CAD build for the part. Positions are in the model's coordinates, mm. A direction names the side the tool comes from. Coordinates: 2 decimals unless noted, no trailing zeros. Loops run counter-clockwise (first coordinate to the right, second up) from the corner with the lowest first, then second, coordinate; pieces in that order, holes last. Notation, with made-up numbers: (-21.75, 82) -> (27.25, 82) arc R28 ccw to (27.25, 118) -> close; hole circle Ø5 at (-38.5, 41.5). An arc over 180 degrees is marked (long way). Write each question's results on one line, items separated by ' | '.
from build123d import *

# Parameters (mm, degrees)
SKETCH1_W           = 200
SKETCH1_H           = 43
BOSS_EXTRUDE1_DEPTH = 25
SKETCH2_W           = 80
SKETCH2_H           = 39
CUT_EXTRUDE1_DEPTH  = 23
SKETCH3_W           = 28
SKETCH3_H           = 14
BOSS_EXTRUDE2_DEPTH = 8
SKETCH4_W           = 14
SKETCH4_H           = 2
BOSS_EXTRUDE3_DEPTH = 2.5
SKETCH5_W           = 14
SKETCH5_H           = 2
BOSS_EXTRUDE4_DEPTH = 2.5
SKETCH6_R           = 1
CUT_EXTRUDE2_DEPTH  = 2
SKETCH7_W           = 116
SKETCH7_H           = 43
CUT_EXTRUDE3_DEPTH  = 23
SKETCH8_W           = 46.953712071
SKETCH8_H           = 43
SKETCH8_R           = 2.1
BOSS_EXTRUDE6_DEPTH = 8
SKETCH9_W           = 10
SKETCH9_H           = 2
CUT_EXTRUDE4_DEPTH  = 61
SKETCH10_W          = 46.769233888
SKETCH10_H          = 43
SKETCH10_R          = 2.1
BOSS_EXTRUDE7_DEPTH = 8
SKETCH11_W          = 3
SKETCH11_H          = 10
CUT_EXTRUDE5_DEPTH  = 8
FILLET1_R           = 15
FILLET2_R           = 15


with BuildPart() as part:
    # Sketch1 → Boss-Extrude1 (new body)
    with BuildSketch(Plane(origin=(0, 0, 0), x_dir=(1, 0, 0), z_dir=(0, 1, 0))):
        with Locations((100, 21.5)):
            Rectangle(SKETCH1_W, SKETCH1_H)
    extrude(amount=BOSS_EXTRUDE1_DEPTH)

    # Sketch2 → Cut-Extrude1 (cut)
    with BuildSketch(Plane(origin=(0, 25, 0), x_dir=(1, 0, 0), z_dir=(0, 1, 0))):
        with Locations((42, 21.5)):
            Rectangle(SKETCH2_W, SKETCH2_H)
    extrude(amount=-CUT_EXTRUDE1_DEPTH, mode=Mode.SUBTRACT)

    # Sketch3 → Boss-Extrude2 (add)
    with BuildSketch(Plane.XZ):
        with Locations((25.914586037, -21)):
            Rectangle(SKETCH3_W, SKETCH3_H)
    extrude(amount=BOSS_EXTRUDE2_DEPTH)

    # Sketch4 → Boss-Extrude3 (add)
    with BuildSketch(Plane(origin=(39.914586037, 0, 0), x_dir=(0, 0, -1), z_dir=(1, 0, 0))):
        with Locations((21, -7)):
            Rectangle(SKETCH4_W, SKETCH4_H)
    extrude(amount=BOSS_EXTRUDE3_DEPTH)

    # Sketch5 → Boss-Extrude4 (add)
    with BuildSketch(Plane.ZY.offset(-11.914586037)):
        with Locations((-21, -7)):
            Rectangle(SKETCH5_W, SKETCH5_H)
    extrude(amount=BOSS_EXTRUDE4_DEPTH)

    # Sketch6 → Cut-Extrude2 (cut)
    with BuildSketch(Plane.XZ):
        with Locations(Location((25.914586037, -37.49, 0), (0, 0, 270))):
            Circle(SKETCH6_R)
        with Locations(Location((28.914586037, -37.49, 0), (0, 0, 270))):
            Circle(SKETCH6_R)
        with Locations(Location((22.914586037, -37.49, 0), (0, 0, 270))):
            Circle(SKETCH6_R)
    extrude(amount=-CUT_EXTRUDE2_DEPTH, mode=Mode.SUBTRACT)

    # Sketch7 → Cut-Extrude3 (cut)
    with BuildSketch(Plane(origin=(0, 25, 0), x_dir=(1, 0, 0), z_dir=(0, 1, 0))):
        with Locations((142, 21.5)):
            Rectangle(SKETCH7_W, SKETCH7_H)
    extrude(amount=-CUT_EXTRUDE3_DEPTH, mode=Mode.SUBTRACT)

    # Sketch8 → Boss-Extrude6 (add)
    with BuildSketch(Plane(origin=(0, 2, 0), x_dir=(1, 0, 0), z_dir=(0, 1, 0))):
        with Locations((176.523143965, 21.5)):
            Rectangle(SKETCH8_W, SKETCH8_H)
        with BuildLine():
            Line((167.769501391, 39.672770255), (184.769501391, 39.672770255))
            Line((184.769501391, 39.672770255), (184.769501391, 34.969828795))
            ThreePointArc((184.769501391, 34.969828795), (187.225820525, 33.318614715), (189.368743796, 31.277073268))
            Line((189.368743796, 31.277073268), (192.70603487, 33.203859168))
            ThreePointArc((192.70603487, 33.203859168), (197.487123783, 31.922770255), (196.20603487, 27.141681341))
            Line((196.20603487, 27.141681341), (192.868743796, 25.214895441))
            ThreePointArc((192.868743796, 25.214895441), (193.542844178, 22.480194155), (193.769501391, 19.672770255))
            ThreePointArc((193.769501391, 19.672770255), (182.474872367, 3.309904642), (163.170258986, 8.068467242))
            Line((163.170258986, 8.068467242), (159.832967911, 6.141681341))
            ThreePointArc((159.832967911, 6.141681341), (155.051878998, 7.422770255), (156.332967911, 12.203859168))
            Line((156.332967911, 12.203859168), (159.670258986, 14.130645068))
            ThreePointArc((159.670258986, 14.130645068), (159.958128459, 26.012258646), (167.769501391, 34.969828795))
            Line((167.769501391, 34.969828795), (167.769501391, 39.672770255))
        make_face(mode=Mode.SUBTRACT)
        with BuildLine():
            Line((192.70603487, 33.203859168), (189.368743796, 31.277073268))
            ThreePointArc((189.368743796, 31.277073268), (191.424945957, 28.422770255), (192.868743796, 25.214895441))
            Line((192.868743796, 25.214895441), (196.20603487, 27.141681341))
            ThreePointArc((196.20603487, 27.141681341), (197.487123783, 31.922770255), (192.70603487, 33.203859168))
        make_face()
        with Locations(Location((194.45603487, 30.172770255, 0), (0, 0, 270))):
            Circle(SKETCH8_R, mode=Mode.SUBTRACT)
        with BuildLine():
            ThreePointArc((163.170258986, 8.068467242), (161.114056824, 10.922770255), (159.670258986, 14.130645068))
            Line((159.670258986, 14.130645068), (156.332967911, 12.203859168))
            ThreePointArc((156.332967911, 12.203859168), (155.051878998, 7.422770255), (159.832967911, 6.141681341))
            Line((159.832967911, 6.141681341), (163.170258986, 8.068467242))
        make_face()
        with Locations(Location((158.082967911, 9.172770255, 0), (0, 0, 270))):
            Circle(SKETCH8_R, mode=Mode.SUBTRACT)
    extrude(amount=BOSS_EXTRUDE6_DEPTH)

    # Sketch9 → Cut-Extrude4 (cut)
    with BuildSketch(Plane.XY):
        with Locations((13, 24)):
            Rectangle(SKETCH9_W, SKETCH9_H)
        with Locations((71, 24)):
            Rectangle(SKETCH9_W, SKETCH9_H)
    extrude(amount=-CUT_EXTRUDE4_DEPTH, mode=Mode.SUBTRACT)

    # Sketch10 → Boss-Extrude7 (add)
    with BuildSketch(Plane(origin=(0, 2, 0), x_dir=(1, 0, 0), z_dir=(0, 1, 0))):
        with Locations((120.116777129, 21.5)):
            Rectangle(SKETCH10_W, SKETCH10_H)
        with BuildLine():
            Line((111.703601521, 39.593697937), (128.703601521, 39.593697937))
            Line((128.703601521, 39.593697937), (128.703601521, 34.890756478))
            ThreePointArc((128.703601521, 34.890756478), (131.159920655, 33.239542397), (133.302843926, 31.19800095))
            Line((133.302843926, 31.19800095), (136.640135, 33.12478685))
            ThreePointArc((136.640135, 33.12478685), (141.421223914, 31.843697937), (140.140135, 27.062609024))
            Line((140.140135, 27.062609024), (136.802843926, 25.135823124))
            ThreePointArc((136.802843926, 25.135823124), (137.476944308, 22.401121838), (137.703601521, 19.593697937))
            ThreePointArc((137.703601521, 19.593697937), (126.408972497, 3.230832325), (107.104359116, 7.989394924))
            Line((107.104359116, 7.989394924), (103.767068041, 6.062609024))
            ThreePointArc((103.767068041, 6.062609024), (98.985979128, 7.343697937), (100.267068041, 12.12478685))
            Line((100.267068041, 12.12478685), (103.604359116, 14.051572751))
            ThreePointArc((103.604359116, 14.051572751), (103.892228589, 25.933186329), (111.703601521, 34.890756478))
            Line((111.703601521, 34.890756478), (111.703601521, 39.593697937))
        make_face(mode=Mode.SUBTRACT)
        with BuildLine():
            Line((136.640135, 33.12478685), (133.302843926, 31.19800095))
            ThreePointArc((133.302843926, 31.19800095), (135.359046087, 28.343697937), (136.802843926, 25.135823124))
            Line((136.802843926, 25.135823124), (140.140135, 27.062609024))
            ThreePointArc((140.140135, 27.062609024), (141.421223914, 31.843697937), (136.640135, 33.12478685))
        make_face()
        with Locations(Location((138.390135, 30.093697937, 0), (0, 0, 270))):
            Circle(SKETCH10_R, mode=Mode.SUBTRACT)
        with BuildLine():
            ThreePointArc((107.104359116, 7.989394924), (105.048156955, 10.843697937), (103.604359116, 14.051572751))
            Line((103.604359116, 14.051572751), (100.267068041, 12.12478685))
            ThreePointArc((100.267068041, 12.12478685), (98.985979128, 7.343697937), (103.767068041, 6.062609024))
            Line((103.767068041, 6.062609024), (107.104359116, 7.989394924))
        make_face()
        with Locations(Location((102.017068041, 9.093697937, 0), (0, 0, 270))):
            Circle(SKETCH10_R, mode=Mode.SUBTRACT)
    extrude(amount=BOSS_EXTRUDE7_DEPTH)

    # Sketch11 → Cut-Extrude5 (cut)
    with BuildSketch(Plane(origin=(84, 0, 0), x_dir=(0, 0, -1), z_dir=(1, 0, 0))):
        with Locations((13.721629554, 17.383252488)):
            Rectangle(SKETCH11_W, SKETCH11_H)
        with Locations((7.721629554, 17.383252488)):
            Rectangle(SKETCH11_W, SKETCH11_H)
    extrude(amount=-CUT_EXTRUDE5_DEPTH, mode=Mode.SUBTRACT)

    # Fillet1
    fillet1_edges = [part.edges().sort_by_distance(p)[0] for p in [
        (200, 5, 0),
    ]]
    fillet(fillet1_edges, radius=FILLET1_R)

    # Fillet2
    fillet2_edges = [part.edges().sort_by_distance(p)[0] for p in [
        (200, 5, -43),
    ]]
    fillet(fillet2_edges, radius=FILLET2_R)


solid = part.part
1) Slice it at C-C (x = 123). Write the cut outline in (y, z).
Outcome:
outline: (0, -43) -> (10, -43) -> (10, -39.59) -> (2, -39.59) -> (2, -2.32) -> (10, -2.32) -> (10, 0) -> (0, 0) -> close
2) Drill centre lines: L1, parallel to Z at x = 83.5, y = 19; L2, parallel to X at y = 0.6, z = -37.49; L3, parallel to X at y = 18.5, z = -35. Where is each one in solid material? Low to high. Write a range as from..to.
Outcome:
L1: z = -43..-15.22, -12.22..-9.22, -6.22..0 | L2: x = 0..21.91, 23.91..24.91, 26.91..27.91, 29.91..196.62 | L3: x = 0..2, 82..84
3) Slice it at B-B (y = -3.5). Write the cut outline in (x, z), then the cut area to 3 significant figures.
Outcome:
outline: (11.91, -28) -> (39.91, -28) -> (39.91, -14) -> (11.91, -14) -> close | area: 392 mm^2
4) Slice it at A-A (y = 19.5). Write the cut outline in (x, z).
Outcome:
outline: (0, -43) -> (84, -43) -> (84, -15.22) -> (82, -15.22) -> (82, -41) -> (2, -41) -> (2, -2) -> (82, -2) -> (82, -6.22) -> (84, -6.22) -> (84, 0) -> (0, 0) -> close; (82, -12.22) -> (84, -12.22) -> (84, -9.22) -> (82, -9.22) -> close
5) Which spindle directions (+Z, -Z, +X, -X, +Y, -Y) get a long thin tool onto all of the face, cutting with end or side? Do faces 4 (the flat face through (90, 2, -22)), 5 (the flat face through (26, -4, -28)), 6 (the flat face through (41, 2, -22)). Say none if no direction does.
Outcome:
face 4: +Z, -Z, +Y | face 5: -Z, +X, -X, -Y | face 6: +Y
6) Pin check, flat tips, straight feed: pin 1 (3 mm diameter, centred on x = 41, z = -20, fed in from +Y); pin 2 (2 mm diameter, centred on x = 158, z = -23.5, fed in from +Y); pin 3 (5 mm diameter, centred on y = 7.5, z = -38, fed in from +X); pin 4 (5 mm diameter, centred on x = 110.5, y = -4.5, fed in from -Z). Stop position of each tip, or through.
Outcome:
pin 1: stops at y = 2 | pin 2: stops at y = 10 | pin 3: stops at x = 197.99 | pin 4: passes through
7) Two-plate mould, pull along Z, no slides. Class faces 1 (the flat face through (153.046, 6, -21)), 2 (the flat face through (41, 14, -2)), 3 (the flat face through (71, 10, 0)): pulls with the +Z half, pulls with the -Z half, needs draft (parallel to the pull), parting line crosses it, or undercut.
Outcome:
face 1: needs draft | face 2: undercut | face 3: pulls with the +Z half
